Here's how the part is built. I have some questions about the finished solid (model axes, mm). Face numbers are marked on the shaded views. Give positions to 0.01 mm unless a question says otherwise; leave off trailing zeros. Loops run counter-clockwise (first coordinate to the right, second up) from the corner with the lowest first, then second, coordinate; pieces in that order, holes last.
Q1. I need wall thicknesses on probe 1 along X at (y, z) = (0, -0.3); probe 2 along Y at (x, z) = (0, -0.25); probe 3 along Z at (x, y) = (0.5, -8). Which ranges of each line are inside material? Lowest first, please.
Q2. Suppose I cut it at C-C (z = 0.6). List the corners of the cut face in (x, y) for me.
Q3. I'm going to push a flat-ended pin straight in: P1, Ø7, axis at x = 15.75, y = 0, coming from the +Z side. Where does the tip first touch, or does it pass through?
Q4. Suppose I cut it at A-A (y = 0). List the corners of the cut face in (x, z) for me, and give its area (4 significant figures).
Q5. Suppose I cut it at D-D (x = 8.5). List the corners of the cut face in (y, z) for me, and give its area (3 significant figures).
Q6. Suppose I cut it at B-B (x = 2). List the corners of the cut face in (y, z) for me.
Q7. Thinking about a two-plate mould opening in X: for the marked faces 1 and 2, which applies, pulls with the +X half, pulls with the -X half, needs draft (parallel to the pull), parting line crosses it, or undercut?
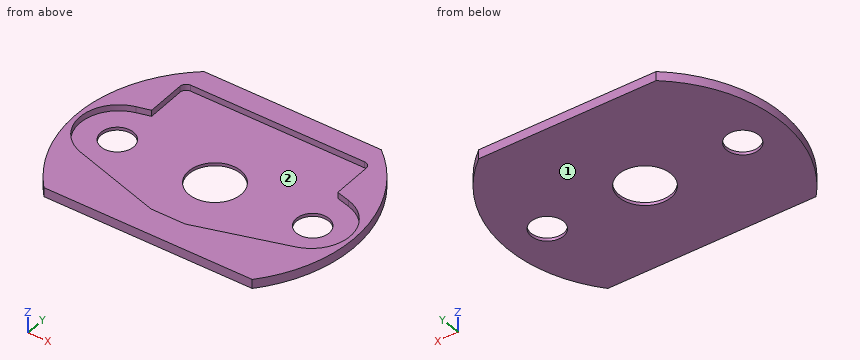
```python
from build123d import *

# Parameters (mm, degrees)
SKETCH_R        = 22.5
PAD_DEPTH       = 1
SKETCH001_R     = 22.5
PAD001_DEPTH    = 0.5
SKETCH002_R     = 4.25
SKETCH002_R_2   = 2.65
POCKET_DEPTH    = 1.501
FILLET_R        = 1
FILLET001_R     = 1
POCKET001_DEPTH = 5


with BuildPart() as part:
    # Sketch → Pad (new body)
    with BuildSketch(Plane.XY):
        Circle(SKETCH_R)
        with BuildLine():
            ThreePointArc((17.347253, -6.023093), (21.799021, 0.111063), (17.133775, 6.08447))
            Line((15, 6.657422), (17.133775, 6.08447))
            Line((15, 14), (15, 6.657422))
            Line((-15, 14), (15, 14))
            Line((-15, 14), (-15, 6.657422))
            Line((-17.133775, 6.08447), (-15, 6.657422))
            ThreePointArc((-17.133775, 6.08447), (-21.799021, 0.111063), (-17.347253, -6.023093))
            Line((-17.347253, -6.023093), (-2.75, -10.5))
            Line((-2.75, -10.5), (2.75, -10.5))
            Line((17.347253, -6.023093), (2.75, -10.5))
        make_face(mode=Mode.SUBTRACT)
    extrude(amount=PAD_DEPTH)

    # Sketch001 (on Face12 of Pad) → Pad001 (join)
    with BuildSketch(Plane(origin=(0, 0, 0), x_dir=(1, 0, 0), z_dir=(0, 0, -1))):
        Circle(SKETCH001_R)
    extrude(amount=PAD001_DEPTH)

    # Sketch002 (on Face4 of Pad001) → Pocket (cut, through all)
    with BuildSketch(Plane(origin=(0, 0, -0.5), x_dir=(1, 0, 0), z_dir=(0, 0, -1))):
        Circle(SKETCH002_R)
        with Locations((-15.75, 0)):
            Circle(SKETCH002_R_2)
        with Locations((15.75, 0)):
            Circle(SKETCH002_R_2)
    extrude(amount=-POCKET_DEPTH, mode=Mode.SUBTRACT)

    # Fillet
    fillet_edges = [part.edges().sort_by_distance(p)[0] for p in [
        (15, 14, 0.5),
        (-15, 14, 0.5),
    ]]
    fillet(fillet_edges, radius=FILLET_R)

    # Fillet001
    fillet001_edges = [part.edges().sort_by_distance(p)[0] for p in [
        (-2.75, -10.5, 0.5),
        (2.75, -10.5, 0.5),
    ]]
    fillet(fillet001_edges, radius=FILLET001_R)

    # Sketch003 (on Face1 of Fillet001) → Pocket001 (cut)
    with BuildSketch(Plane.XY.offset(1)):
        with BuildLine():
            Line((-14.299143, 17.371946), (14.299143, 17.371946))
            ThreePointArc((14.299143, 17.371946), (0, 22.5), (-14.299143, 17.371946))
        make_face()
        with BuildLine():
            Line((16.788655, -14.979688), (-16.788655, -14.979688))
            ThreePointArc((-16.788655, -14.979688), (0, -22.5), (16.788655, -14.979688))
        make_face()
    extrude(amount=-POCKET001_DEPTH, mode=Mode.SUBTRACT)


solid = part.part
```
Solutions:
1. probe 1: x = -22.5 to -18.4, -13.1 to -4.25, 4.25 to 13.1, 18.4 to 22.5
1. probe 2: y = -14.98 to -4.25, 4.25 to 17.37
1. probe 3: z = -0.5 to 0
2. outline: (-16.79, -14.98) - (16.79, -14.98) arc R22.5 ccw to (14.3, 17.37) - (-14.3, 17.37) arc R22.5 ccw to start; hole (-17.35, -6.02) - (-2.89, -10.46) arc R1 ccw to (-2.6, -10.5) - (2.6, -10.5) arc R1 ccw to (2.89, -10.46) - (17.35, -6.02) arc R6.3 ccw to (17.13, 6.08) - (15, 6.66) - (15, 13) arc R1 ccw to (14, 14) - (-14, 14) arc R1 ccw to (-15, 13) - (-15, 6.66) - (-17.13, 6.08) arc R6.3 ccw to start
3. P1: stops at z = 0
4. outline: (-22.5, -0.5) - (-18.4, -0.5) - (-18.4, 0) - (-21.8, 0) - (-21.8, 1) - (-22.5, 1) - close; (-13.1, -0.5) - (-4.25, -0.5) - (-4.25, 0) - (-13.1, 0) - close; (4.25, -0.5) - (13.1, -0.5) - (13.1, 0) - (4.25, 0) - close; (18.4, -0.5) - (22.5, -0.5) - (22.5, 1) - (21.8, 1) - (21.8, 0) - (18.4, 0) - close
4. area: 14.35 mm2
5. outline: (-14.98, -0.5) - (17.37, -0.5) - (17.37, 1) - (14, 1) - (14, 0) - (-8.74, 0) - (-8.74, 1) - (-14.98, 1) - close
5. area: 25.8 mm2
6. outline: (-14.98, -0.5) - (-3.75, -0.5) - (-3.75, 0) - (-10.5, 0) - (-10.5, 1) - (-14.98, 1) - close; (3.75, -0.5) - (17.37, -0.5) - (17.37, 1) - (14, 1) - (14, 0) - (3.75, 0) - close
7. face 1: needs draft
7. face 2: undercut
